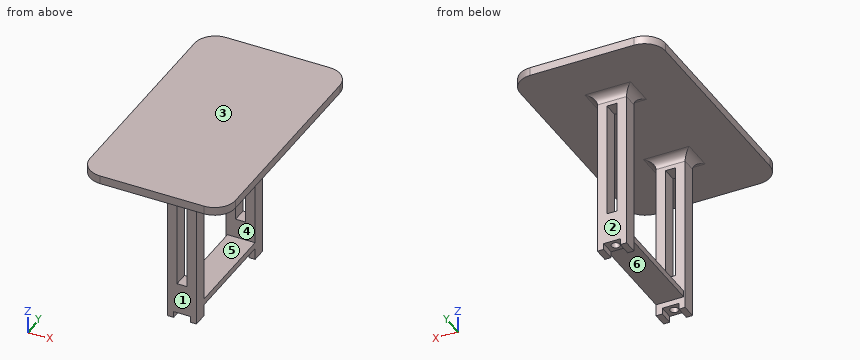
Autodesk Fusion 360 part; units mm, degrees
sketch "Sketch1" plane through (0, 0, 0) normal (0, 0, 1) x (1, 0, 0)
  line L0 (-3.5, -2.6546) -> (3.5, -2.6546)
  line L1 (3.5, -2.6546) -> (3.5, 0.8454)
  line L2 (3.5, 0.8454) -> (-3.5, 0.8454)
  line L3 (-3.5, 0.8454) -> (-3.5, -2.6546)
  circle A0 centre (0, -0.9046) radius 1
  line L4 (-6.5474, 12.8454) -> (3.4526, 12.8454) construction
  line L5 (-3.5, 28.3454) -> (3.5, 28.3454)
  line L6 (-3.5, 24.8454) -> (-3.5, 28.3454)
  circle A1 centre (0, 26.5954) radius 1
  line L7 (3.5, 28.3454) -> (3.5, 24.8454)
  line L8 (3.5, 24.8454) -> (-3.5, 24.8454)
  line L9 (-2, 0.8454) -> (2, 0.8454)
  line L10 (2, 0.8454) -> (2, -2.6546)
  line L11 (2, -2.6546) -> (-2, -2.6546)
  line L12 (-2, -2.6546) -> (-2, 0.8454)
  line L13 (-2, 0.8454) -> (2, -2.6546) construction
  line L14 (2, 0.8454) -> (-2, -2.6546) construction
  line L15 (-2, 28.3454) -> (-2, 24.8454)
  line L16 (2, 24.8454) -> (2, 28.3454)
  line L17 (2, 28.3454) -> (-2, 28.3454)
  line L18 (-2, 24.8454) -> (2, 24.8454)
  point P0 (0, 0.8454)
  point P1 (3.5, -0.9046)
  point P2 (3.5, 26.5954)
  point P3 (0, 24.8454)
  point P4 (0, 25.6909)
  point P5 (0, -0.9046)
  dimension "d1" = 2
  dimension "d2" = 3.5
  dimension "d3" = 7
  dimension "d4" = 10
  dimension "d5" = 12
  dimension "d30" = 4
extrude "Extrude1" add sketch "Sketch1" along normal blind 40 contours L0 L2 L3 L12 | L0 L2 L9 L10 L11 L12 | L0 L1 L2 L10 | A0 | L5 L6 L8 L15 | L5 L8 L15 L16 L17 L18 | L5 L7 L8 L16 | A1 makes body 1 at (1.1667, 0.8454, 13.3333) makes body 2 at (-1.1667, 28.3454, 13.3333)
extrude "Extrude2" cut sketch "Sketch1" along normal blind 8 contours A0 | A1 bodies 1 2
sketch "Sketch2" plane through (0, 0.8454, 0) normal (0, 1, 0) x (-1, 0, 0)
  line L0 (-3.5, 0) -> (3.5, 0)
  line L1 (3.5, 0) -> (3.5, 40)
  line L2 (3.5, 40) -> (-3.5, 40)
  line L3 (-3.5, 40) -> (-3.5, 0)
  line L4 (-1.2, 37) -> (1.2, 37)
  line L5 (1.2, 37) -> (1.2, 9)
  line L6 (1.2, 9) -> (-1.2, 9)
  line L7 (-1.2, 9) -> (-1.2, 37)
  line L8 (3.5, 0) -> (-3.5, 0)
  dimension "d10" = 2.3
  dimension "d11" = 2.3
  dimension "d12" = 9
  dimension "d13" = 3
extrude "Extrude3" cut sketch "Sketch2" along normal through all and the other way through all contours L4 L5 L6 L7 bodies 2
sketch "Sketch3" plane through (0, 0, 0) normal (0, 0, 1) x (1, 0, 0)
  line L0 (17.5, -16.6546) -> (-17.5, -16.6546)
  line L1 (-17.5, -16.6546) -> (-17.5, 42.3454)
  line L2 (-17.5, 42.3454) -> (17.5, 42.3454)
  line L3 (17.5, 42.3454) -> (17.5, -16.6546)
  line L4 (-3.5, -2.6546) -> (3.5, -2.6546)
  line L5 (-3.5, 0.8454) -> (-3.5, -2.6546)
  line L6 (-3.5, 28.3454) -> (3.5, 28.3454)
  line L7 (-4, -16.6546) -> (4, -16.6546)
  line L8 (4, -16.6546) -> (4, -34.6546)
  line L9 (4, -34.6546) -> (-4, -34.6546)
  line L10 (-4, -34.6546) -> (-4, -16.6546)
  line L11 (-4, 42.3454) -> (4, 42.3454)
  line L12 (4, 42.3454) -> (4, 60.3454)
  line L13 (4, 60.3454) -> (-4, 60.3454)
  line L14 (-4, 60.3454) -> (-4, 42.3454)
  line L15 (17.5, 8.8454) -> (35.5, 8.8454)
  line L16 (35.5, 8.8454) -> (35.5, 16.8454)
  line L17 (35.5, 16.8454) -> (17.5, 16.8454)
  line L18 (17.5, 16.8454) -> (17.5, 8.8454)
  line L19 (-17.5, 8.8454) -> (-35.5, 8.8454)
  line L20 (-35.5, 8.8454) -> (-35.5, 16.8454)
  line L21 (-35.5, 16.8454) -> (-17.5, 16.8454)
  line L22 (-17.5, 16.8454) -> (-17.5, 8.8454)
  point P0 (3.5, -0.9046)
  point P1 (0, -34.6546)
  point P2 (-35.5, 12.8454)
  point P3 (35.5, 12.8454)
  point P4 (0, 60.3454)
  point P5 (-17.5, 12.8454)
  dimension "d15" = 14
  dimension "d16" = 14
  dimension "d17" = 14
  dimension "d18" = 14
  dimension "d43" = 8
  dimension "d44" = 18
extrude "Extrude4" add sketch "Sketch3" along normal blind 2 from surface at 40 contours L0 L1 L2 L3 L7 L11 L18 L22 bodies 1 2
fillet "Fillet1" radius 5 4 edges at (-17.5, -16.6546, 41) (-17.5, 42.3454, 41) (17.5, 42.3454, 41) (17.5, -16.6546, 41) on bodies 1
fillet "Fillet1" radius 2 8 edges at (0, 28.3454, 40) (-3.5, 26.5954, 40) (3.5, 26.5954, 40) (0, 24.8454, 40) (3.5, -0.9046, 40) (0, -2.6546, 40) (-3.5, -0.9046, 40) (0, 0.8454, 40) on bodies 1
extrude "Extrude5" cut sketch "Sketch2" against normal blind 8 contours L4 L5 L6 L7 bodies 1
extrude "Extrude6" cut sketch "Sketch1" along normal blind 1.5 contours L0 L2 L9 L10 L11 L12 | L5 L8 L15 L16 L17 L18 bodies 1
sketch "Sketch4" plane through (0, 24.8454, 0) normal (0, -1, 0) x (1, 0, 0)
  line L0 (-1.2, 9) -> (-1.2, 37)
  line L1 (-1.2, 37) -> (1.2, 37)
  line L2 (1.2, 37) -> (1.2, 9)
  line L3 (1.2, 9) -> (-1.2, 9)
  line L4 (-2, 0) -> (-2, 1.5)
  line L5 (-2, 1.5) -> (2, 1.5)
  line L6 (2, 1.5) -> (2, 0)
  line L7 (2, 0) -> (3.5, 0)
  line L8 (3.5, 0) -> (3.5, 38)
  line L9 (3.5, 38) -> (-3.5, 38)
  line L10 (-3.5, 38) -> (-3.5, 0)
  line L11 (-3.5, 0) -> (-2, 0)
  line L12 (3.5, 4.35) -> (-3.5, 4.35)
  line L13 (-3.5, 4.35) -> (-3.5, 2.85)
  line L14 (-3.5, 2.85) -> (3.5, 2.85)
  line L15 (3.5, 2.85) -> (3.5, 4.35)
  line L16 (-3.5, 2.85) -> (-3.1607, 2.85)
  line L17 (-3.1607, 2.85) -> (-3.1607, 4.35)
  line L18 (-3.1607, 4.35) -> (-3.5, 4.35)
  line L19 (-3.5, 4.35) -> (-3.5, 2.85)
  point P0 (3.5, 0)
  dimension "d40" = 1.5
  dimension "d42" = 2.85
extrude "Extrude7" add sketch "Sketch4" along normal up to surface (24 mm away) contours L8 L12 L14 L15 L17 bodies 1
equation "d11 = d10"
equation "d16 = d15"
equation "d17 = d16"
equation "d18 = d15"
equation "d40 = d34"
Could you check a few things on this model? Use its own coordinates, in mm. Face numbers are marked on the shaded views. A direction names the side the tool comes from. Round coordinates to 2 decimals unless told otherwise and drop trailing zeros. Loops run counter-clockwise (first coordinate to the right, second up) from the corner with the lowest first, then second, coordinate; pieces in that order, holes last. Notation, with made-up numbers: (69.5, 76.5) - (107.5, 76.5) arc R15 ccw to (107.5, 92.5) - close; hole circle Ø5 at (89.25, 55). An arc over 180 degrees is marked (long way). Write item = value, one per line.
1) Imagine slicing it at A-A (z = 6.5). Please give me the cut outline in (x, y).
Computed:
outline = (-3.5, -2.65) - (3.5, -2.65) - (3.5, 0.85) - (-3.5, 0.85) - close; (-3.5, 24.85) - (3.5, 24.85) - (3.5, 28.35) - (-3.5, 28.35) - close; hole circle Ø2 at (0, -0.9); hole circle Ø2 at (0, 26.6)
2) I need wall thicknesses on line 1 along Y through (x, z) = (0, 6.75); line 2 along Z through (x, y) = (-2, 12.5); line 3 along Y through (x, z) = (3, 19). Which ranges of each line are inside material? Lowest first, please. Write a range as from..to.
Computed:
line_1 = -2.65..-1.9, 0.1..0.85, 24.85..25.6, 27.6..28.35
line_2 = 2.85..4.35, 40..42
line_3 = -2.65..0.85, 24.85..28.35
3) I'm going to push flat-ended pins straight in: P1, Ø3, axis at y = -1, z = 22.5, coming from the -X side; P2, Ø0.6, axis at x = 0, y = 27, coming from the -Z side; P3, Ø3, axis at x = -4.5, z = 23, coming from the -Y side. Where does each tip first touch, or does it pass through?
Computed:
P1 = -3.5
P2 = 8
P3 = -2.65
4) If we mould it in two halves opening along Z, with no side actions, what happens to the marked faces 3, 4, 5 and 6? For each: pulls with the +Z half, pulls with the -Z half, needs draft (parallel to the pull), parting line crosses it, or undercut.
Computed:
face_3 = pulls with the +Z half
face_4 = undercut
face_5 = undercut
face_6 = pulls with the -Z half
5) Imagine slicing it at C-C (z = 27.5). Please give me the cut outline in (x, y).
Computed:
outline = (-3.5, -2.65) - (-1.2, -2.65) - (-1.2, 0.85) - (-3.5, 0.85) - close; (-3.5, 24.85) - (-1.2, 24.85) - (-1.2, 28.35) - (-3.5, 28.35) - close; (1.2, -2.65) - (3.5, -2.65) - (3.5, 0.85) - (1.2, 0.85) - close; (1.2, 24.85) - (3.5, 24.85) - (3.5, 28.35) - (1.2, 28.35) - close
6) Imagine slicing it at B-B (y = 19). Please give me the cut outline in (x, z), and give its area (3 significant figures).
Computed:
outline = (-17.5, 40) - (17.5, 40) - (17.5, 42) - (-17.5, 42) - close; (-3.16, 2.85) - (3.5, 2.85) - (3.5, 4.35) - (-3.16, 4.35) - close
area = 80.0 mm2
7) On a 3-axis mill with a long thin cutter (end or side, diameter ignored), from which of +Z, -Z, +X, -X, +Y, -Y can I reach the whole of each face in a straight line? I mean the marked faces 1 and 2. Say none if no direction works.
Computed:
face_1 = -Z, +X, -X, -Y
face_2 = -Z, +X, -X, +Y
8) Imagine slicing it at D-D (z = 39). Please give me the cut outline in (x, y), and give its area (3 significant figures).
Computed:
outline = (-3.77, -2.92) - (3.77, -2.92) - (3.77, 1.11) - (-3.77, 1.11) - close; (-3.77, 24.58) - (3.77, 24.58) - (3.77, 28.61) - (-3.77, 28.61) - close
area = 60.8 mm2
